from build123d import *

# Parameters (mm, degrees)
SKETCH2_W               = 254
SKETCH2_H               = 101.6
BOSS_EXTRUDE1_DEPTH     = 4.7625
FILLET1_R               = 6.35
F_6_CLEARANCE_HOLE1_D   = 3.7973
F_1_4_CLEARANCE_HOLE1_D = 6.7564


with BuildPart() as part:
    # Sketch2 → Boss-Extrude1 (new body)
    with BuildSketch(Plane(origin=(0, 0, 0), x_dir=(1, 0, 0), z_dir=(0, 1, 0))):
        with Locations((127, -50.8)):
            Rectangle(SKETCH2_W, SKETCH2_H)
    extrude(amount=BOSS_EXTRUDE1_DEPTH)

    # Fillet1
    fillet1_edges = [part.edges().sort_by_distance(p)[0] for p in [
        (0, 2.38125, 0),
        (254, 2.38125, 0),
        (254, 2.38125, 101.6),
        (0, 2.38125, 101.6),
    ]]
    fillet(fillet1_edges, radius=FILLET1_R)

    # #6 Clearance Hole1 (through all)
    with Locations(Plane(origin=(0, 4.7625, 0), x_dir=(1, 0, 0), z_dir=(0, 1, 0))):
        with Locations((66.675, -25.4), (187.325, -25.4)):
            Hole(F_6_CLEARANCE_HOLE1_D / 2)

    # 1/4 Clearance Hole1 (through all)
    with Locations(Plane(origin=(0, 4.7625, 0), x_dir=(1, 0, 0), z_dir=(0, 1, 0))):
        with Locations((12.7, -12.7), (12.7, -88.9), (241.3, -88.9), (241.3, -12.7), (12.7, -50.8), (241.3, -50.8)):
            Hole(F_1_4_CLEARANCE_HOLE1_D / 2)


solid = part.part
Model file for the job. Use its own axes, mm. Coordinates: 2 decimals unless noted, no trailing zeros. Write each loop counter-clockwise with the first axis right and the second up, starting at its lowest first coordinate (ties: lowest second). Pieces come first, ordered by that corner, then holes. Notation, with made-up numbers: (76, 17.25) - (122, 17.25) arc R30 ccw to (122, 54.25) - close; hole circle Ø3 at (65, 74.5). An arc over 180 degrees is marked (long way). Write each question's results on one line, items separated by ' | '. Start each with the question number.
1) Probe line 1 along X through (y, z) = (1.9, 88.9); line 2 along Z through (x, y) = (239, 0.3); line 3 along X through (y, z) = (1.9, 87). List the from-to ranges inside material, lowest first. Write a range as from..to.
2) Mould opens along Z. For faces 1 (the face through (125, 2, 0)), 2 (the face through (125, 4.762, 50)), 3 (the face through (244.675, 2.348, 12.551)), 4 (the face through (1.81, 2.41, 99.69)) say: pulls with the +Z half, pulls with the -Z half, needs draft (parallel to the pull), parting line crosses it, or undercut.
3) Cut at B-B (x = 241.3). Write the cut outline in (y, z).
4) Flat gauge pin, fed straight in: P1, Ø6, axis at x = 127.5, z = 86.5, coming from the -Y side. Where does the tip first touch, or does it go through?
5) Cut at A-A (z = 88.9). Write the cut outline in (x, y), then the cut area to 3 significant figures.
Returned:
1) line 1: 0..9.32, 16.08..237.92, 244.68..254 | line 2: 0..10.23, 15.17..48.33, 53.27..86.43, 91.37..101.6 | line 3: 0..9.91, 15.49..238.51, 244.09..254
2) face 1: pulls with the -Z half | face 2: needs draft | face 3: undercut | face 4: pulls with the +Z half
3) outline: (0, 0) - (4.76, 0) - (4.76, 9.32) - (0, 9.32) - close; (0, 16.08) - (4.76, 16.08) - (4.76, 47.42) - (0, 47.42) - close; (0, 54.18) - (4.76, 54.18) - (4.76, 85.52) - (0, 85.52) - close; (0, 92.28) - (4.76, 92.28) - (4.76, 101.6) - (0, 101.6) - close
4) P1: y = 0
5) outline: (0, 0) - (9.32, 0) - (9.32, 4.76) - (0, 4.76) - close; (16.08, 0) - (237.92, 0) - (237.92, 4.76) - (16.08, 4.76) - close; (244.68, 0) - (254, 0) - (254, 4.76) - (244.68, 4.76) - close | area: 1,150 mm^2
